Source: CAD feature listing. Evaluate the final solid. Frame: model axes, mm. A direction names the side the tool comes from. Give positions to 0.01 mm unless a question says otherwise; leave off trailing zeros. Order: outer loops, then holes, each group sorted by start corner. A loop starts at its lowest first (then second) coordinate and runs counter-clockwise, first axis right, second up.
1) Access query for faces 1 (the face through (96.961, -38, 23)), 2 (the face through (137, -59.726, 5)), 3 (the face through (41, -104.14, 28)), 4 (the face through (47, -38.1, 89)). Directions: +Z, -Z, +X, -X, +Y, -Y. A direction counts if a zero-diameter tool reaches every point of the face in a straight line with its end or side. Return the directions, or none.
2) Section B-B, the plane x = 281. Return loops of the section in (y, z).
3) Draft query along Y for faces 5 (the face through (171, -111, 0)), 6 (the face through (47, 0, 26)), 7 (the face through (143, -37, 0)). Return one class per face: released by +Y, released by -Y, zero draft, split by the parting line, or undercut.
4) Section C-C, the plane y = 56. Return loops of the section in (x, z), plus the area to 3 significant figures.
5) First-contact query: P1, Ø5.5, axis at x = 37.5, z = 24.5, coming from the -Y side; P2, Ø2, axis at x = 31, y = -102.5, coming from the +Z side; P3, Ø2, axis at y = -31.5, z = 14.5, coming from the +X side. Flat tips, straight axial feed; report the tip coordinate or a pass-through.
6) Section A-A, the plane z = 29. Return loops of the section in (x, y).
7) Section D-D, the plane y = 132. Return loops of the section in (x, z), plus the area to 3 significant figures.
8) Material intervals for line 1 (Y direction, x = 0, z = -6); line 2 (X direction, y = -99.5, z = 2), sorted ascending.
```python
from build123d import *

# Parameters (mm, degrees)
F0_W      = 94.4209545851
F0_H      = 76.6059160233
F1_DEPTH  = 101.6
F2_SIZE   = 25.4
F3_W      = 25.4
F3_H      = 25.4
F4_DEPTH  = 25.4
F6_W      = 45.1313219965
F6_H      = 6.7916600965
F7_DEPTH  = 101.6
F5_W      = 63.737494871
F5_H      = 17.642442137
F8_DEPTH  = 2.54
F9_W      = 43.406561017
F9_H      = 32.155352179
F10_DEPTH = 2.54
F11_W     = 690.3821974993
F11_H     = 486.4143431187
F12_DEPTH = 76.2
F14_R     = 156.1146532665
F15_DEPTH = 25.4
F16_R     = 134.4660155787
F17_DEPTH = 25.4


with BuildPart() as f1:
    # F0 (on Front) → F1 (new body)
    with BuildSketch(Plane.XZ):
        with Locations((47.2104772925, 38.3029580116)):
            Rectangle(F0_W, F0_H)
    extrude(amount=F1_DEPTH)

    # F2
    f2_edges = [f1.edges().sort_by_distance(p)[0] for p in [
        (94.420955, -50.8, 76.605916),
        (0, -50.8, 76.605916),
        (47.210477, 0, 76.605916),
        (47.210477, -101.6, 76.605916),
    ]]
    chamfer(f2_edges, length=F2_SIZE)

    # F3 (on face) → F4 (join)
    with BuildSketch(Plane.XY.offset(76.6059160233)):
        with Locations((47.1932, -50.8)):
            Rectangle(F3_W, F3_H)
    extrude(amount=F4_DEPTH)

    # F6 (on face) → F7 (join)
    with BuildSketch(Plane.YZ.offset(94.4209545851)):
        with Locations((-37.1608156711, 3.3958300482)):
            Rectangle(F6_W, F6_H)
    extrude(amount=F7_DEPTH)

    # F5 (on face) → F8 (join)
    with BuildSketch(Plane.XZ.offset(101.6)):
        with Locations((41.0035112873, 27.7578178793)):
            Rectangle(F5_W, F5_H)
    extrude(amount=F8_DEPTH)

    # F9 (on face) → F10 (join)
    with BuildSketch(Plane.YZ.offset(94.4209545851)):
        with Locations((-38.0231961608, 22.869336186)):
            Rectangle(F9_W, F9_H)
    extrude(amount=F10_DEPTH)

    # F11 (on face) → F12 (join)
    with BuildSketch(Plane(origin=(0, 0, 0), x_dir=(1, 0, 0), z_dir=(0, 0, -1))):
        with Locations((99.6137782931, 53.9849847555)):
            Rectangle(F11_W, F11_H)
        Polygon((0, 0), (0, 101.6), (94.4209545851, 101.6), (94.4209545851, 59.7264766693), (196.0209545851, 59.7264766693), (196.0209545851, 14.5951546729), (94.4209545851, 14.5951546729), (94.4209545851, 0), align=None, mode=Mode.SUBTRACT)
        Polygon((94.4209545851, 101.6), (0, 101.6), (0, 0), (94.4209545851, 0), (94.4209545851, 14.5951546729), (196.0209545851, 14.5951546729), (196.0209545851, 59.7264766693), (94.4209545851, 59.7264766693), align=None)
    extrude(amount=F12_DEPTH)

    # F14 (on face) → F15 (cut)
    with BuildSketch(Plane.XY):
        with Locations((0, -36.4867895842)):
            Circle(F14_R)
    extrude(amount=-F15_DEPTH, mode=Mode.SUBTRACT)

    # F16 (on face) → F17 (join, through all)
    with BuildSketch(Plane.XY):
        with Locations((0, -27.1963328123)):
            Circle(F16_R)
    extrude(amount=-F17_DEPTH)


solid = f1.part
```
From the geometry:
1. face 1: +Z, +X, +Y, -Y
1. face 2: +Z, +X, -Y
1. face 3: +Z, +X, -X, -Y
1. face 4: +Z, +X, -X, +Y
2. outline: (-297.19, -76.2) - (189.22, -76.2) - (189.22, 0) - (-297.19, 0) - close
3. face 5: zero draft
3. face 6: released by +Y
3. face 7: undercut
4. outline: (-245.58, -76.2) - (444.8, -76.2) - (444.8, 0) - (125.77, 0) - (125.77, -25.4) - (105.64, -25.4) - (105.64, 0) - (-105.64, 0) - (-105.64, -25.4) - (-125.77, -25.4) - (-125.77, 0) - (-245.58, 0) - close
4. area: 51,600 mm2
5. P1: stops at y = -104.14
5. P2: stops at z = 51.31
5. P3: stops at x = 96.96
6. outline: (0, -101.6) - (9.13, -101.6) - (9.13, -104.14) - (72.87, -104.14) - (72.87, -101.6) - (94.42, -101.6) - (94.42, -59.73) - (96.96, -59.73) - (96.96, -16.32) - (94.42, -16.32) - (94.42, 0) - (0, 0) - close
7. outline: (-245.58, -76.2) - (444.8, -76.2) - (444.8, 0) - (-245.58, 0) - close
7. area: 52,600 mm2
8. line 1: y = -297.19 to -192.6, -161.66 to 107.27, 119.63 to 189.22
8. line 2: x = 0 to 94.42
